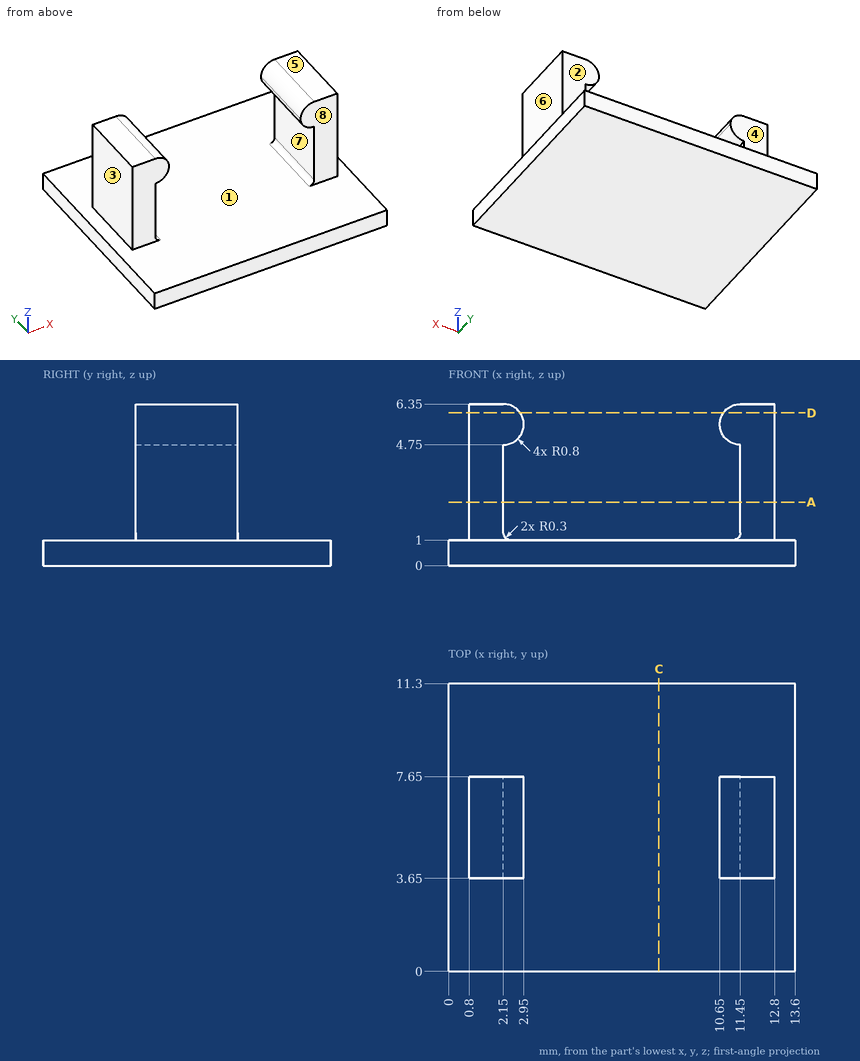
Input: dimensioned drawing with shaded views. Units: mm. Origin: part minimum x, y, z. A direction names the side the tool comes from. Round coordinates to 2 decimals unless told otherwise and drop trailing zeros. Order: outer loops, then holes, each group sorted by start corner. A loop starts at its lowest first (then second) coordinate and runs counter-clockwise, first axis right, second up. Notation, with made-up numbers: (85.5, -33.75) -> (101.5, -33.75) arc R25 ccw to (101.5, -16.75) -> close; hole circle Ø3 at (-32, 18.5). An arc over 180 degrees is marked (long way). Put each result on its own line as item: value. Start each with the question number.
Q1. Section A-A on z = 2.5. Return the cut outline in (x, y).
Q2. Reachability of the marked faces 4, 5, 6, 7 and 8 from +Z, -Z, +X, -X, +Y, -Y: full face, straight path, thin tool, end or side. Return the list, or none.
Q3. Line query: probe 1 along X at (y, z) = (6.5, 2); probe 2 along Z at (x, y) = (9.25, 8.25); probe 3 along Z at (x, y) = (2.5, 7.5). Output: solid intervals per line, ascending.
Q4. Section D-D on z = 6. Return the cut outline in (x, y), and give its area (3 significant figures).
Q5. First-contact query: pin 1 (2 mm diameter, centred on y = 5.5, z = 4, fed in from -X); pin 2 (3 mm diameter, centred on y = 5, z = 4, fed in from +X); pin 3 (3 mm diameter, centred on x = 6.5, y = 4, fed in from +Z). Flat tips, straight axial feed; report the tip coordinate or a pass-through.
Q6. Section C-C on x = 8.25. Return the cut outline in (y, z), and give its area (3 significant figures).
Q7. Pull-direction query (X, two-part tool) for the marked faces 1, 2 and 3; classes: +X half, -X half, draft (parallel to the pull), parting line (faces both ways), or undercut.
Ans:
1. outline: (0.8, 3.65) -> (2.15, 3.65) -> (2.15, 7.65) -> (0.8, 7.65) -> close; (11.45, 3.65) -> (12.8, 3.65) -> (12.8, 7.65) -> (11.45, 7.65) -> close
2. face 4: +Z, +X, -X, +Y
2. face 5: +Z, +X, -X, +Y, -Y
2. face 6: +Z, +X, +Y, -Y
2. face 7: +Y, -Y
2. face 8: +Z, +X, -X, -Y
3. probe 1: x = 0.8 to 2.15, 11.45 to 12.8
3. probe 2: z = 0 to 1
3. probe 3: z = 0 to 1, 4.83 to 6.27
4. outline: (0.8, 3.65) -> (2.81, 3.65) -> (2.81, 7.65) -> (0.8, 7.65) -> close; (10.79, 3.65) -> (12.8, 3.65) -> (12.8, 7.65) -> (10.79, 7.65) -> close
4. area: 16.1 mm2
5. pin 1: stops at x = 0.8
5. pin 2: stops at x = 12.8
5. pin 3: stops at z = 1
6. outline: (0, 0) -> (11.3, 0) -> (11.3, 1) -> (0, 1) -> close
6. area: 11.3 mm2
7. face 1: undercut
7. face 2: draft
7. face 3: -X half
